from build123d import *

# Parameters (mm, degrees)
SKETCH1_W               = 6.485
SKETCH1_H               = 4.5
BOSS_EXTRUDE1_DEPTH     = 88
BOSS_EXTRUDE1_2_DEPTH   = 88
SKETCH3_W               = 2
SKETCH3_H               = 1.5
CUT_EXTRUDE2_DEPTH      = 30
SKETCH4_W               = 2
SKETCH4_H               = 4.5
CUT_EXTRUDE3_DEPTH      = 65
BOSS_EXTRUDE2_REACH     = 93.644
SKETCH6_W               = 67
SKETCH6_H               = 3
BOSS_EXTRUDE3_DEPTH     = 5
CUT_EXTRUDE4_DEPTH      = 5
BOSS_EXTRUDE4_DEPTH     = 5
BOSS_EXTRUDE5_START     = 7
BOSS_EXTRUDE5_DEPTH     = 48
BOSS_EXTRUDE6_DEPTH     = 48
FILLET1_R               = 11
SKETCH15_W              = 23.7
SKETCH15_H              = 21.22267295
CUT_EXTRUDE6_DEPTH      = 7
SKETCH16_W              = 16.7
SKETCH16_H              = 1.5
CUT_EXTRUDE7_DEPTH      = 19
CUT_EXTRUDE5_DEPTH      = 92.727000479
CUT_EXTRUDE5_DEPTH_BACK = 92.727000479
SKETCH13_R              = 1.5


with BuildPart() as part:
    # Sketch1 → Boss-Extrude1 (new body)
    with BuildSketch(Plane.XY):
        with Locations((-11.5925, 2.25)):
            Rectangle(SKETCH1_W, SKETCH1_H)
    extrude(amount=-BOSS_EXTRUDE1_DEPTH)


with BuildPart() as body_2:
    # Sketch1 → Boss-Extrude1 2 (new body)
    with BuildSketch(Plane.XY):
        with Locations((11.5925, 2.25)):
            Rectangle(SKETCH1_W, SKETCH1_H)
    extrude(amount=-BOSS_EXTRUDE1_2_DEPTH)


with BuildPart() as cut_extrude2_tool:
    # Sketch3 → Cut-Extrude2 (new body)
    with BuildSketch(Plane.XY):
        with Locations((-9.35, 0.75)):
            Rectangle(SKETCH3_W, SKETCH3_H)
        with Locations((9.35, 0.75)):
            Rectangle(SKETCH3_W, SKETCH3_H)
    extrude(amount=-CUT_EXTRUDE2_DEPTH)


with BuildPart() as part_1:
    add(part.part)

    # Cut-Extrude2: cut by cut_extrude2_tool
    add(cut_extrude2_tool.part, mode=Mode.SUBTRACT)


with BuildPart() as body_2_1:
    add(body_2.part)

    # Cut-Extrude2: cut by cut_extrude2_tool
    add(cut_extrude2_tool.part, mode=Mode.SUBTRACT)


with BuildPart() as cut_extrude3_tool:
    # Sketch4 → Cut-Extrude3 (new body)
    with BuildSketch(Plane(origin=(0, 0, -88), x_dir=(-1, 0, 0), z_dir=(0, 0, -1))):
        with Locations((9.35, 2.25)):
            Rectangle(SKETCH4_W, SKETCH4_H)
        with Locations((-9.35, 2.25)):
            Rectangle(SKETCH4_W, SKETCH4_H)
    extrude(amount=-CUT_EXTRUDE3_DEPTH)


with BuildPart() as part_2:
    add(part_1.part)

    # Cut-Extrude3: cut by cut_extrude3_tool
    add(cut_extrude3_tool.part, mode=Mode.SUBTRACT)


with BuildPart() as body_2_2:
    add(body_2_1.part)

    # Cut-Extrude3: cut by cut_extrude3_tool
    add(cut_extrude3_tool.part, mode=Mode.SUBTRACT)

    # Boss-Extrude2: up to this face of the body (flat: up to its plane)
    boss_extrude2_end = Plane(body_2_2.part.faces().sort_by_distance((10.35, 2.091743119, -50.857798165))[0])
    # Sketch6 → Boss-Extrude2 (add, up to the picked face)
    with BuildSketch(Plane(origin=(-10.35, 0, 0), x_dir=(0, 0, -1), z_dir=(1, 0, 0)), mode=Mode.PRIVATE) as boss_extrude2_sk1:
        with Locations((49.5, 3)):
            Rectangle(SKETCH6_W, SKETCH6_H)
    boss_extrude2_tool1 = split(extrude(boss_extrude2_sk1.sketch, amount=BOSS_EXTRUDE2_REACH, mode=Mode.PRIVATE), bisect_by=boss_extrude2_end, keep=Keep.BOTH, mode=Mode.PRIVATE)

    add(part_2.part)  # Boss-Extrude2 merges part
    add(boss_extrude2_tool1.solids().sort_by(Axis((-10.35, 3, -49.5), (1, 0, 0)))[0])

    # Sketch8 → Boss-Extrude3 (add)
    with BuildSketch(Plane(origin=(0, 0, -88), x_dir=(-1, 0, 0), z_dir=(0, 0, -1))):
        Polygon((-14.835, 25.70767295), (-14.835, 4.5), (-10.35, 4.5), (-10.35, 21.22267295), (10.35, 21.22267295), (10.35, 4.5), (14.835, 4.5), (14.835, 25.70767295), align=None)
    extrude(amount=-BOSS_EXTRUDE3_DEPTH)

    # Sketch9 → Cut-Extrude4 (cut)
    with BuildSketch(Plane(origin=(0, 0, -88), x_dir=(-1, 0, 0), z_dir=(0, 0, -1))):
        with BuildLine():
            Line((-15.009070225, 25.881743175), (-15.009070225, 22.527310239))
            ThreePointArc((-15.009070225, 22.527310239), (-13.436955933, 24.309628883), (-11.654637289, 25.881743175))
            Line((-11.654637289, 25.881743175), (-15.009070225, 25.881743175))
        make_face()
        with BuildLine():
            Line((15.009070225, 25.881743175), (15.009070225, 22.527310239))
            ThreePointArc((15.009070225, 22.527310239), (13.436955933, 24.309628883), (11.654637289, 25.881743175))
            Line((11.654637289, 25.881743175), (15.009070225, 25.881743175))
        make_face()
    extrude(amount=-CUT_EXTRUDE4_DEPTH, mode=Mode.SUBTRACT)

    # Sketch11 → Boss-Extrude4 (add)
    with BuildSketch(Plane.XY.offset(-83)):
        with BuildLine():
            Line((14.835, 4.5), (14.835, 22.748097759))
            ThreePointArc((14.835, 22.748097759), (13.436955933, 24.309628883), (11.875424809, 25.70767295))
            Line((11.875424809, 25.70767295), (-11.875424809, 25.70767295))
            ThreePointArc((-11.875424809, 25.70767295), (-13.436955933, 24.309628883), (-14.835, 22.748097759))
            Line((-14.835, 22.748097759), (-14.835, 4.5))
            Line((-14.835, 4.5), (14.835, 4.5))
        make_face()
    extrude(amount=BOSS_EXTRUDE4_DEPTH)

    # Sketch12 → Boss-Extrude5 (add)
    with BuildSketch(Plane.XY.offset(-78).offset(BOSS_EXTRUDE5_START)):
        Polygon((-14.835, 4.5), (-11.835, 7.5), (11.835, 7.5), (14.835, 4.5), align=None)
    extrude(amount=BOSS_EXTRUDE5_DEPTH)

    # Sketch14 → Boss-Extrude6 (add)
    with BuildSketch(Plane.XY.offset(-23)):
        Polygon((-11.835, 7.5), (-14.835, 4.5), (-10.835, 4.5), (-10.835, 7.5), align=None)
        Polygon((11.835, 7.5), (14.835, 4.5), (10.835, 4.5), (10.835, 7.5), align=None)
    extrude(amount=-BOSS_EXTRUDE6_DEPTH)

    # Fillet1
    # the kernel refuses this fillet: 11 mm, written as the material it takes off along each edge
    with BuildSketch(Plane(origin=(11.835, 7.5, -82.374586088), x_dir=(-1, 0, 0), z_dir=(0, 0, 1))) as fillet1_piece_1_section:
        with BuildLine():
            CenterArc((4.549834435, 11), FILLET1_R, 226.658241773, 43.341758227)
            Line((-3, 3), (0, 0))
            Line((0, 0), (4.549834435, 0))
        make_face()
    fillet1_piece_1 = extrude(amount=70.749172176, mode=Mode.PRIVATE)
    fillet1_piece_1 = split(fillet1_piece_1, bisect_by=Plane(origin=(11.355308805, 6.742969198, -78), z_dir=(0, 0, 1)), keep=Keep.TOP, mode=Mode.PRIVATE)
    add(fillet1_piece_1, mode=Mode.SUBTRACT)
    with BuildSketch(Plane(origin=(-11.835, 7.5, -82.374586088), x_dir=(1, 0, 0), z_dir=(0, 0, 1))) as fillet1_piece_2_section:
        with BuildLine():
            CenterArc((4.549834435, -11), FILLET1_R, 90, 43.341758227)
            Line((-3, -3), (0, 0))
            Line((0, 0), (4.549834435, 0))
        make_face()
    fillet1_piece_2 = extrude(amount=70.749172176, mode=Mode.PRIVATE)
    fillet1_piece_2 = split(fillet1_piece_2, bisect_by=Plane(origin=(-11.355308805, 6.742969198, -78), z_dir=(0, 0, 1)), keep=Keep.TOP, mode=Mode.PRIVATE)
    add(fillet1_piece_2, mode=Mode.SUBTRACT)

    # Sketch15 → Cut-Extrude6 (cut)
    with BuildSketch(Plane(origin=(0, 0, -88), x_dir=(-1, 0, 0), z_dir=(0, 0, -1))):
        with Locations((0, 12.111336475)):
            Rectangle(SKETCH15_W, SKETCH15_H)
    extrude(amount=-CUT_EXTRUDE6_DEPTH, mode=Mode.SUBTRACT)

    # Sketch16 → Cut-Extrude7 (cut)
    with BuildSketch(Plane.XY):
        with BuildLine():
            ThreePointArc((11.5925, 3.75), (10.014054255, 3.189942939), (8.35, 3))
            Line((8.35, 3), (8.35, 4.5))
            Line((8.35, 4.5), (14.835, 4.5))
            ThreePointArc((14.835, 4.5), (13.170945745, 4.310057061), (11.5925, 3.75))
        make_face()
        with BuildLine():
            ThreePointArc((-11.5925, 3.75), (-10.014054255, 3.189942939), (-8.35, 3))
            Line((-8.35, 3), (-8.35, 4.5))
            Line((-8.35, 4.5), (-14.835, 4.5))
            ThreePointArc((-14.835, 4.5), (-13.170945745, 4.310057061), (-11.5925, 3.75))
        make_face()
        with Locations((0, 3.75)):
            Rectangle(SKETCH16_W, SKETCH16_H)
    extrude(amount=-CUT_EXTRUDE7_DEPTH, mode=Mode.SUBTRACT)

    # Sketch13 → Cut-Extrude5 (cut, two sides: drawn at the far end of the back side and taken through both)
    with BuildSketch(Plane(origin=(0, 4.5, 0), x_dir=(1, 0, 0), z_dir=(0, 1, 0)).offset(-CUT_EXTRUDE5_DEPTH_BACK)):
        with Locations(Location((10.542662348, 74.5, 0), (0, 0, 97.379545614))):
            Circle(SKETCH13_R)
        with Locations(Location((-10.542662348, 74.5, 0), (0, 0, 277.379545614))):
            Circle(SKETCH13_R)
        with Locations(Location((10.542662348, 21, 0), (0, 0, 97.379545614))):
            Circle(SKETCH13_R)
        with Locations(Location((-10.542662348, 21, 0), (0, 0, 277.379545614))):
            Circle(SKETCH13_R)
    extrude(amount=CUT_EXTRUDE5_DEPTH + CUT_EXTRUDE5_DEPTH_BACK, mode=Mode.SUBTRACT)


solid = body_2_2.part
Build history of the part. All positions in model axes, mm. A direction names the side the tool comes from. Round coordinates to 2 decimals unless told otherwise and drop trailing zeros. Write each loop counter-clockwise with the first axis right and the second up, starting at its lowest first coordinate (ties: lowest second). Pieces come first, ordered by that corner, then holes. Notation, with made-up numbers: (10, 38) - (49, 38) arc R8 cw to (49, 48) - close; hole circle Ø7 at (10, 56). An arc over 180 degrees is marked (long way). One line per question, with ' | ' between items.
1. Band-saw the part on A-A, the plane z = -74.5. Write the cut outline in (x, y) (3 decimals).
Results are:
outline: (-14.835, 0) - (-12.043, 0) - (-12.043, 4.5) - (-14.835, 4.5) - close; (-9.043, 1.5) - (9.043, 1.5) - (9.043, 4.5) - (-9.043, 4.5) - close; (12.043, 0) - (14.835, 0) - (14.835, 4.5) - (12.043, 4.5) - close
2. Mould opens along X. For faces 4 (the face through (0, 4.5, -74)), 5 (the face through (-11.293, 6.744, -47.336)), 6 (the face through (11, 1.5, -85)) say: released by +X, released by -X, zero draft, split by the parting line, or undercut.
Results are:
face 4: zero draft | face 5: released by -X | face 6: undercut
3. Tool access for faces 1 (the face through (10.35, 1, -10)), 2 (the face through (0, 7.5, -47)), 3 (the face through (0, 12, -81)): list every direction of +Z, -Z, +X, -X, +Y, -Y with a clear straight run to the whole face (end or side of a thin tool).
Results are:
face 1: +Z, -Z, -Y | face 2: +Z, +X, -X, +Y | face 3: -Z
4. Drill centre lines: line 1 along X through (y, z) = (1.75, -74.5) (3 decimals); line 2 along X through (y, z) = (1.3, -74.5) (3 decimals); line 3 along Z through (x, y) = (-9.25, 3.5). Where is each one in solid material? Low to high. Write a range as from..to.
Results are:
line 1: -14.835..-12.043, -9.043..9.043, 12.043..14.835 | line 2: -14.835..-12.043, 12.043..14.835 | line 3: -81..-75.26, -73.74..-21.76, -20.24..-19
5. Drop flat-ended pins along their axis: pin 1 Ø3.5 at (x, z) = (6, -86) entering from -Y; pin 2 Ø3.5 at (x, z) = (-10.54, -21) entering from +Y; pin 3 Ø1 at (x, z) = (-5, -68) entering from -Y. Give the stop position or say it passes through.
Results are:
pin 1: y = 22.72 | pin 2: y = 4.5 | pin 3: y = 1.5
6. Band-saw the part on B-B, the plane x = 0. Write the cut outline in (y, z).
Results are:
outline: (1.5, -81) - (22.72, -81) - (22.72, -88) - (25.71, -88) - (25.71, -78) - (4.5, -78) - (4.5, -71) - (7.5, -71) - (7.5, -23) - (4.5, -23) - (4.5, -19) - (3, -19) - (3, -16) - (1.5, -16) - close
7. Band-saw the part on D-D, the plane z = -54. Write the cut outline in (x, y) (3 decimals).
Results are:
outline: (-14.835, 0) - (-10.35, 0) - (-10.35, 1.5) - (10.35, 1.5) - (10.35, 0) - (14.835, 0) - (14.835, 4.5) arc R11 ccw to (7.285, 7.5) - (-7.285, 7.5) arc R11 ccw to (-14.835, 4.5) - close
